The model under review builds one solid part; all positions refer to its coordinate system, in mm. A direction names the side the tool comes from. Round coordinates to 2 decimals unless told otherwise and drop trailing zeros. Loops run counter-clockwise (first coordinate to the right, second up) from the corner with the lowest first, then second, coordinate; pieces in that order, holes last. Notation, with made-up numbers: M 20,-38 L 61,-38 A32 ccw 61,-12 Z; hole C 73.25,77 d6. An arc over 180 degrees is marked long. Return JSON: item names as keys, results as strings. Group by question number.
Q1. Clearance check with flat-ended pins moving along their axes: pin 1 Ø5 at (x, z) = (12.5, -6) entering from +Y; pin 2 Ø3.5 at (x, y) = (0, 15) entering from +Z; pin 3 Ø4.5 at (x, y) = (0, 15) entering from -Z. State where each tip first meets the part, or that it passes through.
Q2. Consider section C-C (y = 18.75). State the section outline as (x, z) points.
Q3. Draft analysis for pull direction X (two halves, no side actions). For faces 4 (the face through (19.34, 14.08, -19.55)), 5 (the face through (17, 8, -6)), 6 (the face through (-23.3, 13, 0)), 7 (the face through (13.31, 3.45, -6.08)), state which applies: pulls with the +X half, pulls with the -X half, needs draft (parallel to the pull), parting line crosses it, or undercut.
Q4. Consider section A-A (y = 9). State the section outline as (x, z) points.
Q5. To check wall thickness, follow line 1 along Z through (x, y) = (7, 15.5); line 2 along Z through (x, y) = (0, 4.5); line 3 along Y through (x, z) = (0, -21.1). State the ranges of each line that lie inside material, in increasing order.
Q6. Consider section B-B (z = -6.75). State the section outline as (x, y) points.
Q7. Consider section D-D (x = 22). State the section outline as (y, z) points.
Q8. For faces 1 (the face through (-0.228, 3.451, 11.765)), 2 (the face through (24.314, 12.267, 0.607)), 3 (the face through (-16.158, 14.93, -16.015)), list the 3-axis set-ups (+Z, -Z, +X, -X, +Y, -Y) from which the entire face can be reached by the end or side of a thin tool; tool diameter is ignored.
from build123d import *

# Parameters (mm, degrees)
SKETCH_1_R           = 17.5
SKETCH_1_R_2         = 1.75
EXTRUDE_1_DEPTH      = 10
SKETCH_2_R           = 25
SKETCH_2_R_2         = 17.5
EXTRUDE_2_DEPTH      = 2
SKETCH_3_R           = 3.25
CUT_EXTRUDE_1_DEPTH  = 3
EXTRUDE_3_DEPTH      = 10
EXTRUDE_3_DEPTH_BACK = 2
SKETCH_6_R           = 1.65
CUT_EXTRUDE_2_DEPTH  = 54.5
SKETCH_7_R           = 1.65
CUT_EXTRUDE_3_DEPTH  = 54.5
SKETCH_8_R           = 2.8
CUT_EXTRUDE_4_DEPTH  = 2
SKETCH_9_R           = 2.8
CUT_EXTRUDE_5_DEPTH  = 2
SKETCH_10_R          = 2.8
CUT_EXTRUDE_6_DEPTH  = 2
SKETCH_11_R          = 2.8
CUT_EXTRUDE_7_DEPTH  = 2


with BuildPart() as part:
    # 草图1 → 凸台-拉伸1 (new body)
    with BuildSketch(Plane(origin=(0, 0, 0), x_dir=(1, 0, 0), z_dir=(0, 1, 0))):
        Circle(SKETCH_1_R)
        with Locations((0, 13.5)):
            Circle(SKETCH_1_R_2, mode=Mode.SUBTRACT)
        with Locations((11.691342951, 6.75)):
            Circle(SKETCH_1_R_2, mode=Mode.SUBTRACT)
        with Locations((11.691342951, -6.75)):
            Circle(SKETCH_1_R_2, mode=Mode.SUBTRACT)
        with Locations((0, -13.5)):
            Circle(SKETCH_1_R_2, mode=Mode.SUBTRACT)
        with Locations((-11.691342951, -6.75)):
            Circle(SKETCH_1_R_2, mode=Mode.SUBTRACT)
        with Locations((-11.691342951, 6.75)):
            Circle(SKETCH_1_R_2, mode=Mode.SUBTRACT)
    extrude(amount=EXTRUDE_1_DEPTH)

    # 草图2 → 凸台-拉伸2 (add)
    with BuildSketch(Plane(origin=(0, 10, 0), x_dir=(1, 0, 0), z_dir=(0, 1, 0))):
        Circle(SKETCH_2_R)
        Circle(SKETCH_2_R_2, mode=Mode.SUBTRACT)
    extrude(amount=-EXTRUDE_2_DEPTH)

    # 草图3 → 切除-拉伸1 (cut)
    with BuildSketch(Plane(origin=(0, 10, 0), x_dir=(1, 0, 0), z_dir=(0, 1, 0))):
        with Locations((0, 13.5)):
            Circle(SKETCH_3_R)
        with Locations((11.691342951, 6.75)):
            Circle(SKETCH_3_R)
        with Locations((11.691342951, -6.75)):
            Circle(SKETCH_3_R)
        with Locations((0, -13.5)):
            Circle(SKETCH_3_R)
        with Locations((-11.691342951, -6.75)):
            Circle(SKETCH_3_R)
        with Locations((-11.691342951, 6.75)):
            Circle(SKETCH_3_R)
    extrude(amount=-CUT_EXTRUDE_1_DEPTH, mode=Mode.SUBTRACT)

    # 草图4 → 凸台-拉伸3 (add, two sides)
    with BuildSketch(Plane(origin=(0, 10, 0), x_dir=(1, 0, 0), z_dir=(0, 1, 0))) as extrude_3_sk:
        with BuildLine():
            Line((-10.777754868, 25.3), (10.777754868, 25.3))
            ThreePointArc((10.777754868, 25.3), (19.445436483, 19.445436483), (25.3, 10.777754868))
            Line((25.3, 10.777754868), (25.3, -10.777754868))
            ThreePointArc((25.3, -10.777754868), (19.445436483, -19.445436483), (10.777754868, -25.3))
            Line((10.777754868, -25.3), (-10.777754868, -25.3))
            ThreePointArc((-10.777754868, -25.3), (-19.445436483, -19.445436483), (-25.3, -10.777754868))
            Line((-25.3, -10.777754868), (-25.3, 10.777754868))
            ThreePointArc((-25.3, 10.777754868), (-19.445436483, 19.445436483), (-10.777754868, 25.3))
        make_face()
        with BuildLine():
            Line((-10.269980526, 20.3), (10.269980526, 20.3))
            ThreePointArc((10.269980526, 20.3), (16.086679272, 16.086679272), (20.3, 10.269980526))
            Line((20.3, 10.269980526), (20.3, -10.269980526))
            ThreePointArc((20.3, -10.269980526), (16.086679272, -16.086679272), (10.269980526, -20.3))
            Line((10.269980526, -20.3), (-10.269980526, -20.3))
            ThreePointArc((-10.269980526, -20.3), (-16.086679272, -16.086679272), (-20.3, -10.269980526))
            Line((-20.3, -10.269980526), (-20.3, 10.269980526))
            ThreePointArc((-20.3, 10.269980526), (-16.086679272, 16.086679272), (-10.269980526, 20.3))
        make_face(mode=Mode.SUBTRACT)
    extrude(amount=EXTRUDE_3_DEPTH)
    extrude(extrude_3_sk.sketch, amount=-EXTRUDE_3_DEPTH_BACK)

    # 草图6 → 切除-拉伸2 (cut, symmetric)
    with BuildSketch(Plane.XY.offset(25.3)):
        with Locations((0, 15)):
            Circle(SKETCH_6_R)
    extrude(amount=CUT_EXTRUDE_2_DEPTH, both=True, mode=Mode.SUBTRACT)

    # 草图7 → 切除-拉伸3 (cut, symmetric)
    with BuildSketch(Plane(origin=(25.3, 0, 0), x_dir=(0, 0, -1), z_dir=(1, 0, 0))):
        with Locations((0, 15)):
            Circle(SKETCH_7_R)
    extrude(amount=CUT_EXTRUDE_3_DEPTH, both=True, mode=Mode.SUBTRACT)

    # 草图8 → 切除-拉伸4 (cut)
    with BuildSketch(Plane(origin=(25.3, 0, 0), x_dir=(0, 0, -1), z_dir=(1, 0, 0))):
        with Locations((0, 15)):
            Circle(SKETCH_8_R)
    extrude(amount=-CUT_EXTRUDE_4_DEPTH, mode=Mode.SUBTRACT)

    # 草图9 → 切除-拉伸5 (cut)
    with BuildSketch(Plane(origin=(0, 0, -25.3), x_dir=(-1, 0, 0), z_dir=(0, 0, -1))):
        with Locations((0, 15)):
            Circle(SKETCH_9_R)
    extrude(amount=-CUT_EXTRUDE_5_DEPTH, mode=Mode.SUBTRACT)

    # 草图10 → 切除-拉伸6 (cut)
    with BuildSketch(Plane.ZY.offset(25.3)):
        with Locations((0, 15)):
            Circle(SKETCH_10_R)
    extrude(amount=-CUT_EXTRUDE_6_DEPTH, mode=Mode.SUBTRACT)

    # 草图11 → 切除-拉伸7 (cut)
    with BuildSketch(Plane.XY.offset(25.3)):
        with Locations((0, 15)):
            Circle(SKETCH_11_R)
    extrude(amount=-CUT_EXTRUDE_7_DEPTH, mode=Mode.SUBTRACT)


solid = part.part
Values:
{
 "1": {"pin 1": "stops at y = 10", "pin 2": "stops at z = 23.3", "pin 3": "stops at z = -23.3"},
 "2": {"outline": "M -25.3,-10.78 A27.5 ccw -10.78,-25.3 L 10.78,-25.3 A27.5 ccw 25.3,-10.78 L 25.3,10.78 A27.5 ccw 10.78,25.3 L -10.78,25.3 A27.5 ccw -25.3,10.78 Z; hole M -20.3,-10.27 A22.75 ccw -10.27,-20.3 L 10.27,-20.3 A22.75 ccw 20.3,-10.27 L 20.3,10.27 A22.75 ccw 10.27,20.3 L -10.27,20.3 A22.75 ccw -20.3,10.27 Z"},
 "3": {"face 4": "pulls with the +X half", "face 5": "needs draft", "face 6": "pulls with the -X half", "face 7": "undercut"},
 "4": {"outline": "M -25.3,-10.78 A27.5 ccw -10.78,-25.3 L 10.78,-25.3 A27.5 ccw 25.3,-10.78 L 25.3,10.78 A27.5 ccw 10.78,25.3 L -10.78,25.3 A27.5 ccw -25.3,10.78 Z; hole C -11.69,-6.75 d6.5; hole C -11.69,6.75 d6.5; hole C 0,-13.5 d6.5; hole C 0,13.5 d6.5; hole C 11.69,-6.75 d6.5; hole C 11.69,6.75 d6.5"},
 "5": {"line 1": "z = -25.3 to -20.3, 20.3 to 25.3", "line 2": "z = -17.5 to -15.25, -11.75 to 11.75, 15.25 to 17.5", "line 3": "y = 8 to 13.35, 16.65 to 20"},
 "6": {"outline": "M -25.3,8 L -16.15,8 L -16.15,0 L -13.44,0 L -13.44,7 L -14.94,7 L -14.94,10 L -20.3,10 L -20.3,20 L -25.3,20 Z; M -9.94,0 L 9.94,0 L 9.94,7 L 8.44,7 L 8.44,10 L -8.44,10 L -8.44,7 L -9.94,7 Z; M 13.44,0 L 16.15,0 L 16.15,8 L 25.3,8 L 25.3,20 L 20.3,20 L 20.3,10 L 14.94,10 L 14.94,7 L 13.44,7 Z"},
 "7": {"outline": "M 8,-16.5 L 20,-16.5 L 20,16.5 L 8,16.5 Z; hole C 15,0 d3.3"},
 "8": {"face 1": "+Y, -Y", "face 2": "+X", "face 3": "+Y"}
}
